Could you check a few things on this model? Use its own coordinates, in mm. Face numbers are marked on the shaded views. A direction names the side the tool comes from. Give positions to 0.01 mm unless a question says otherwise; leave off trailing zeros. Loops run counter-clockwise (first coordinate to the right, second up) from the corner with the lowest first, then second, coordinate; pieces in that order, holes last. Notation, with made-up numbers: M 86.25,-23 L 94.25,-23 A32 cw 94.25,12 Z; hole C 27.5,35.25 d5. An arc over 180 degrees is marked long. Use a Markdown table: item, result. Add a question column.
1) Suppose I cut it at B-B on x = 25. List the corners of the cut face in (y, z) for me, and give its area (4 significant figures).
2) Suppose I cut it at C-C on z = 4.2. List the corners of the cut face in (x, y) for me, and give its area (3 significant figures).
3) We'd pull the mould along X, two halves only. Please class the marked faces 3 and 4: +X half, -X half, draft (parallel to the pull), parting line (faces both ways), or undercut.
4) Which directions (+Z, -Z, +X, -X, +Y, -Y) give clear straight access to the entire face, cutting with the end or side of a thin tool? Please do the marked faces 1 and 2.
5) Suppose I cut it at A-A on y = 11.5. List the corners of the cut face in (x, z) for me.
6) Will these pins go through, and if not, where does the flat tip stop? pin 1 Ø2.5 at (y, z) = (13, 3) entering from -X; pin 2 Ø0.8 at (y, z) = (24, 4) entering from -X; pin 3 Ø1.5 at (y, z) = (22.5, 4) entering from +X; pin 4 Ø1.2 at (x, z) = (16, 3.5) entering from -Y.
7) If I drill on line 1 along Y through (x, z) = (15, 3.1); line 2 along Y through (x, z) = (19, 1.25); line 3 along Y through (x, z) = (29.5, 3.35), over which ranges is the centre line in solid material (lowest first)? Write a range as [from, to].
8) Suppose I cut it at D-D on y = 37. List the corners of the cut face in (x, z) for me, and give its area (3 significant figures).
```python
from build123d import *

# Parameters (mm, degrees)
SKETCH1_W           = 40
SKETCH1_H           = 40
BOSS_EXTRUDE2_DEPTH = 2.5
SKETCH2_W           = 30
SKETCH2_H           = 30
BOSS_EXTRUDE3_DEPTH = 2.5
SKETCH3_R           = 1.5
CUT_EXTRUDE1_DEPTH  = 2.5
SKETCH4_W           = 20
SKETCH4_H           = 6
CUT_EXTRUDE2_DEPTH  = 5


with BuildPart() as part:
    # Sketch1 → Boss-Extrude2 (new body)
    with BuildSketch(Plane.XY):
        with Locations((20, 20)):
            Rectangle(SKETCH1_W, SKETCH1_H)
    extrude(amount=BOSS_EXTRUDE2_DEPTH)

    # Sketch2 → Boss-Extrude3 (add)
    with BuildSketch(Plane.XY.offset(2.5)):
        with Locations((20, 20)):
            Rectangle(SKETCH2_W, SKETCH2_H)
    extrude(amount=BOSS_EXTRUDE3_DEPTH)

    # Sketch3 → Cut-Extrude1 (cut)
    with BuildSketch(Plane.XY.offset(2.5)):
        with Locations((3, 37)):
            Circle(SKETCH3_R)
        with Locations((37, 37)):
            Circle(SKETCH3_R)
        with Locations((37, 3)):
            Circle(SKETCH3_R)
        with Locations((3, 3)):
            Circle(SKETCH3_R)
    extrude(amount=-CUT_EXTRUDE1_DEPTH, mode=Mode.SUBTRACT)

    # Sketch4 → Cut-Extrude2 (cut)
    with BuildSketch(Plane.XY.offset(5)):
        Polygon((27.48142397, 31.5), (14.48142397, 31.5), (11.5, 28.833333333), (11.5, 26.333333333), (14.48142397, 23), (27.48142397, 23), align=None)
        with Locations((20, 12)):
            Rectangle(SKETCH4_W, SKETCH4_H)
    extrude(amount=-CUT_EXTRUDE2_DEPTH, mode=Mode.SUBTRACT)


solid = part.part
```
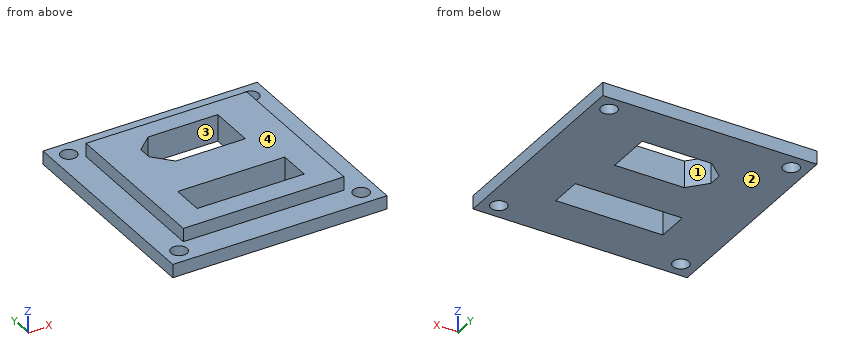
Answer block:
| question | item | result |
|---|---|---|
| 1 | outline | M 0,0 L 9,0 L 9,5 L 5,5 L 5,2.5 L 0,2.5 Z; M 15,0 L 23,0 L 23,5 L 15,5 Z; M 31.5,0 L 40,0 L 40,2.5 L 35,2.5 L 35,5 L 31.5,5 Z |
| 1 | area | 102.5 mm^2 |
| 2 | outline | M 5,5 L 35,5 L 35,35 L 5,35 Z; hole M 10,9 L 30,9 L 30,15 L 10,15 Z; hole M 11.5,26.33 L 14.48,23 L 27.48,23 L 27.48,31.5 L 14.48,31.5 L 11.5,28.83 Z |
| 2 | area | 653 mm^2 |
| 3 | face 3 | undercut |
| 3 | face 4 | draft |
| 4 | face 1 | +Z, -Z |
| 4 | face 2 | -Z, +X, -X, +Y, -Y |
| 5 | outline | M 0,0 L 10,0 L 10,5 L 5,5 L 5,2.5 L 0,2.5 Z; M 30,0 L 40,0 L 40,2.5 L 35,2.5 L 35,5 L 30,5 Z |
| 6 | pin 1 | stops at x = 0 |
| 6 | pin 2 | stops at x = 5 |
| 6 | pin 3 | stops at x = 35 |
| 6 | pin 4 | stops at y = 5 |
| 7 | line 1 | y = [5, 9], [15, 23], [31.5, 35] |
| 7 | line 2 | y = [0, 9], [15, 23], [31.5, 40] |
| 7 | line 3 | y = [5, 9], [15, 35] |
| 8 | outline | M 0,0 L 1.5,0 L 1.5,2.5 L 0,2.5 Z; M 4.5,0 L 35.5,0 L 35.5,2.5 L 4.5,2.5 Z; M 38.5,0 L 40,0 L 40,2.5 L 38.5,2.5 Z |
| 8 | area | 85.0 mm^2 |
